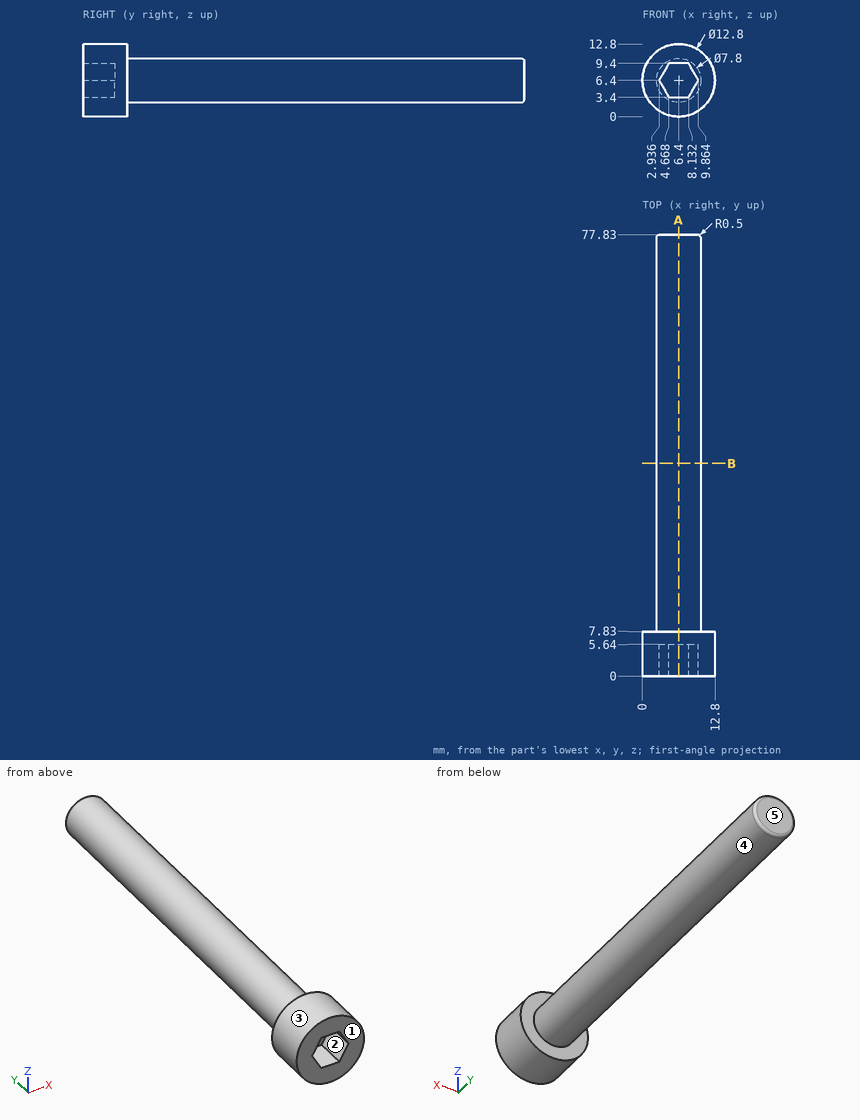
Check sheet for the drawn part. Datum: minimum x, y, z corner. Units: mm. A direction names the side the tool comes from. Coordinates: 2 decimals unless noted, no trailing zeros. Order: outer loops, then holes, each group sorted by start corner. A loop starts at its lowest first (then second) coordinate and runs counter-clockwise, first axis right, second up. Notation, with made-up numbers: (-5.75, 2.25) -> (25.25, 2.25) arc R13 cw to (25.25, 16.25) -> close; hole circle Ø1 at (-15, -18). An arc over 180 degrees is marked (long way). Use a Markdown table: item, result. Add a question column.
1. Material ranges on L1, parallel to Y at x = 10.75, z = 11; L2, parallel to Z at x = 6.75, y = 46; L3, parallel to Z at x = 8.75, y = 57.5, recorded low to high.
2. Go/stop test with flat-tipped pins: pin 1 Ø1.5 at (y, z) = (15, 3.5) entering from -X; pin 2 Ø2 at (x, z) = (1.5, 4) entering from +Y; pin 3 Ø1.5 at (x, z) = (6.5, 6.5) entering from -Y; pin 4 Ø4 at (x, z) = (10.5, 8) entering from -Y. Record where each tip stops, or that it passes through.
3. Set-up check for the marked faces 4 and 5: record each of +Z, -Z, +X, -X, +Y, -Y from which the full face is reachable in a straight line by a thin tool's end or side.
4. Mould release check, pull along X, two halves, no side actions. Record for the marked faces 1, 2 and 3: pulls with the +X half, pulls with the -X half, needs draft (parallel to the pull), parting line crosses it, or undercut.
5. Cross-section at B-B (y = 37.5). Enter the section's corners in (x, z).
6. Cross-section at A-A (x = 6.4). Enter the section's corners in (y, z), and give its area (3 significant figures).
Filled sheet:
| question | item | result |
|---|---|---|
| 1 | L1 | 0 to 7.83 |
| 1 | L2 | 2.52 to 10.28 |
| 1 | L3 | 3.29 to 9.51 |
| 2 | pin 1 | x = 3.15 |
| 2 | pin 2 | y = 7.83 |
| 2 | pin 3 | y = 5.64 |
| 2 | pin 4 | y = 0 |
| 3 | face 4 | +Y |
| 3 | face 5 | +Z, -Z, +X, -X, +Y |
| 4 | face 1 | needs draft |
| 4 | face 2 | undercut |
| 4 | face 3 | parting line crosses it |
| 5 | outline | circle Ø7.8 at (6.4, 6.4) |
| 6 | outline | (0, 0) -> (7.83, 0) -> (7.83, 2.5) -> (77.33, 2.5) arc R0.5 ccw to (77.83, 3) -> (77.83, 9.8) arc R0.5 ccw to (77.33, 10.3) -> (7.83, 10.3) -> (7.83, 12.8) -> (0, 12.8) -> (0, 9.4) -> (5.64, 9.4) -> (5.64, 3.4) -> (0, 3.4) -> close |
| 6 | area | 612 mm2 |
